```python
from build123d import *

# Parameters (mm, degrees)
CROQUIS1_W              = 21
CROQUIS1_H              = 16
CROQUIS1_R              = 1.5
SALIENTE_EXTRUIR1_DEPTH = 1.5
CROQUIS2_R              = 0.55
CORTAR_EXTRUIR1_DEPTH   = 1.5


with BuildPart() as part:
    # Croquis1 → Saliente-Extruir1 (new body)
    with BuildSketch(Plane.XY):
        Rectangle(CROQUIS1_W, CROQUIS1_H)
        with Locations((-8, 5.5)):
            Circle(CROQUIS1_R, mode=Mode.SUBTRACT)
        with Locations(Location((8, 5.5, 0), (0, 0, 180))):
            Circle(CROQUIS1_R, mode=Mode.SUBTRACT)
    extrude(amount=SALIENTE_EXTRUIR1_DEPTH)

    # Croquis2 → Cortar-Extruir1 (cut)
    with BuildSketch(Plane(origin=(0, 0, 0), x_dir=(-1, 0, 0), z_dir=(0, 0, -1))):
        with Locations((-8.75, -6.75)):
            Circle(CROQUIS2_R)
        with Locations((-6.21, -6.75)):
            Circle(CROQUIS2_R)
        with Locations((-3.67, -6.75)):
            Circle(CROQUIS2_R)
        with Locations((-1.13, -6.75)):
            Circle(CROQUIS2_R)
        with Locations((1.41, -6.75)):
            Circle(CROQUIS2_R)
        with Locations((3.95, -6.75)):
            Circle(CROQUIS2_R)
        with Locations((6.49, -6.75)):
            Circle(CROQUIS2_R)
        with Locations((9.03, -6.75)):
            Circle(CROQUIS2_R)
    extrude(amount=-CORTAR_EXTRUIR1_DEPTH, mode=Mode.SUBTRACT)


solid = part.part
```
CAD build for the part. Positions are in the model's coordinates, mm. Give positions to 0.01 mm unless a question says otherwise; leave off trailing zeros. Order: outer loops, then holes, each group sorted by start corner. A loop starts at its lowest first (then second) coordinate and runs counter-clockwise, first axis right, second up.
(1) Saw through at A-A, the plane x = 6.21. Give the cut face in (y, z), then the cut area to 4 significant figures.
(2) Drill centre lines: L1, parallel to Y at x = 8, z = 1.05; L2, parallel to Y at x = -9.25, z = 1.45; L3, parallel to X at y = 6, z = 0.65. Where is each one in solid material? Low to high.
(3) Saw through at C-C, the plane z = 0.7. State how many separate pieces and enclosed holes the cut face has, then the cut area to 3 significant figures.
(4) Mould opens along X. For faces 1 (the flat face through (0, 0, 0)), 2 (the cylindrical face through (-1.291, -7.287, 0.74)), 3 (the flat face through (-10.5, 0, 1)) say: released by +X, released by -X, zero draft, split by the parting line, or undercut.
(5) Saw through at D-D, the plane x = -9.03. Give the cut face in (y, z), then the cut area to 3 significant figures.
(6) Saw through at B-B, the plane y = 5.5. Give the cut face in (x, z), then the cut area to 3 significant figures.
Results found:
1. outline: (-8, 0) - (-7.3, 0) - (-7.3, 1.5) - (-8, 1.5) - close; (-6.2, 0) - (8, 0) - (8, 1.5) - (-6.2, 1.5) - close
1. area: 22.35 mm2
2. L1: y = -8 to 4, 7 to 8
2. L2: y = -8 to -7.25, -6.25 to 4.67, 6.33 to 8
2. L3: x = -10.5 to -9.41, -6.59 to 6.59, 9.41 to 10.5
3. separate pieces: 1
3. enclosed holes: 10
3. area: 314 mm2
4. face 1: zero draft
4. face 2: undercut
4. face 3: released by -X
5. outline: (-8, 0) - (-7.3, 0) - (-7.3, 1.5) - (-8, 1.5) - close; (-6.2, 0) - (4.41, 0) - (4.41, 1.5) - (-6.2, 1.5) - close; (6.59, 0) - (8, 0) - (8, 1.5) - (6.59, 1.5) - close
5. area: 19.1 mm2
6. outline: (-10.5, 0) - (-9.5, 0) - (-9.5, 1.5) - (-10.5, 1.5) - close; (-6.5, 0) - (6.5, 0) - (6.5, 1.5) - (-6.5, 1.5) - close; (9.5, 0) - (10.5, 0) - (10.5, 1.5) - (9.5, 1.5) - close
6. area: 22.5 mm2
